Geometry: final body of the model. Coordinates: model frame, mm. A direction names the side the tool comes from. Coordinates: 2 decimals unless noted, no trailing zeros. Write each loop counter-clockwise with the first axis right and the second up, starting at its lowest first coordinate (ties: lowest second). Pieces come first, ordered by that corner, then holes. Notation, with made-up numbers: (-34.75, 54) - (-11.75, 54) arc R18 cw to (-11.75, 71) - close; hole circle Ø9 at (33, 33). An arc over 180 degrees is marked (long way). Answer as a JSON object with one key per item and string values. Group by question number.
Item 1: Set-up query: faces 1 (the flat face through (4.056, 0, 65)), 2 (the cylindrical face through (-13.5, -0.07, 19.72)). Return all of +Z, -Z, +X, -X, +Y, -Y with unobstructed straight access to the full face (end or side cutting, diameter ignored); none if empty.
Item 2: First-contact query: pin 1 Ø4.5 at (x, y) = (15, 0) entering from -Z; pin 2 Ø2 at (x, y) = (-28.5, 1) entering from +Z; pin 3 Ø4 at (y, z) = (-0.5, 53) entering from -X. Flat tips, straight axial feed; report the tip coordinate or a pass-through.
Item 3: Section C-C on y = 0. State how many separate pieces and enclosed holes the cut face has, and give its area (3 significant figures).
Item 4: Section A-A on x = -37.5. Return loops of the section in (y, z).
Item 5: Mould query, pull axis X, two halves, no side actions, for faces 3 (the flat face through (-1, 2, 0)), 4 (the flat face through (-45, 0, 20)), 5 (the cylindrical face through (-38.226, -1.138, 19.72)), 6 (the cylindrical face through (20.93, 0.65, 44.37)). Classes: pulls with the +X half, pulls with the -X half, needs draft (parallel to the pull), parting line crosses it, or undercut.
Item 6: Section D-D on x = 30. Return loops of the section in (y, z), and give its area (3 significant figures).
Item 7: Section B-B on z = 83. Return loops of the section in (x, y).
Item 8: Line query: line 1 along Y through (x, z) = (29.5, 40.5); line 2 along Y through (x, z) = (0, 29); line 3 along Z through (x, y) = (-25, 0.25). Output: solid intervals per line, ascending. Write a range as from..to.
```python
from build123d import *

# Parameters (mm, degrees)
SKETCH1_W           = 90
SKETCH1_H           = 7.5
SKETCH1_R           = 1.35
SKETCH1_R_2         = 1.4
SKETCH1_R_3         = 1.45
SKETCH1_R_4         = 1.5
SKETCH1_R_5         = 1.6
SKETCH1_R_6         = 1.65
SKETCH1_R_7         = 1.7
SKETCH1_R_8         = 1.8
SKETCH1_R_9         = 1.75
BOSS_EXTRUDE1_DEPTH = 90
SKETCH2_W           = 49.055817317
SKETCH2_H           = 7.5
CUT_EXTRUDE1_DEPTH  = 50


with BuildPart() as part:
    # Sketch1 → Boss-Extrude1 (new body)
    with BuildSketch(Plane.XY):
        Rectangle(SKETCH1_W, SKETCH1_H)
        with Locations(Location((-37.5, 0, 0), (0, 0, 180))):
            Circle(SKETCH1_R, mode=Mode.SUBTRACT)
        with Locations(Location((-30, 0, 0), (0, 0, 180))):
            Circle(SKETCH1_R_2, mode=Mode.SUBTRACT)
        with Locations(Location((-22.5, 0, 0), (0, 0, 180))):
            Circle(SKETCH1_R_3, mode=Mode.SUBTRACT)
        with Locations(Location((-15, 0, 0), (0, 0, 180))):
            Circle(SKETCH1_R_4, mode=Mode.SUBTRACT)
        with Locations(Location((0, 0, 0), (0, 0, 180))):
            Circle(SKETCH1_R_5, mode=Mode.SUBTRACT)
        with Locations(Location((15, 0, 0), (0, 0, 180))):
            Circle(SKETCH1_R_6, mode=Mode.SUBTRACT)
        with Locations(Location((22.5, 0, 0), (0, 0, 180))):
            Circle(SKETCH1_R_7, mode=Mode.SUBTRACT)
        with Locations(Location((37.5, 0, 0), (0, 0, 180))):
            Circle(SKETCH1_R_8, mode=Mode.SUBTRACT)
        with Locations(Location((30, 0, 0), (0, 0, 180))):
            Circle(SKETCH1_R_9, mode=Mode.SUBTRACT)
    extrude(amount=BOSS_EXTRUDE1_DEPTH)

    # Sketch2 → Cut-Extrude1 (cut)
    with BuildSketch(Plane.XY.offset(90)):
        with Locations((-20.472091342, 0)):
            Rectangle(SKETCH2_W, SKETCH2_H)
    extrude(amount=-CUT_EXTRUDE1_DEPTH, mode=Mode.SUBTRACT)


solid = part.part
```
Checks:
{
 "1": {"face 1": "+Z, -X, +Y, -Y", "face 2": "+Z, -Z"},
 "2": {"pin 1": "z = 0", "pin 2": "z = 40", "pin 3": "x = 4.06"},
 "3": {"separate pieces": "10", "enclosed holes": "0", "area": "3,820 mm^2"},
 "4": {"outline": "(-3.75, 0) - (-1.35, 0) - (-1.35, 40) - (-3.75, 40) - close; (1.35, 0) - (3.75, 0) - (3.75, 40) - (1.35, 40) - close"},
 "5": {"face 3": "needs draft", "face 4": "pulls with the -X half", "face 5": "undercut", "face 6": "undercut"},
 "6": {"outline": "(-3.75, 0) - (-1.75, 0) - (-1.75, 90) - (-3.75, 90) - close; (1.75, 0) - (3.75, 0) - (3.75, 90) - (1.75, 90) - close", "area": "360 mm^2"},
 "7": {"outline": "(4.06, -3.75) - (45, -3.75) - (45, 3.75) - (4.06, 3.75) - close; hole circle Ø3.3 at (15, 0); hole circle Ø3.4 at (22.5, 0); hole circle Ø3.5 at (30, 0); hole circle Ø3.6 at (37.5, 0)"},
 "8": {"line 1": "-3.75..-1.68, 1.68..3.75", "line 2": "-3.75..-1.6, 1.6..3.75", "line 3": "0..40"}
}
